from build123d import *

# Parameters (mm, degrees)
SKETCH20_R          = 3.817056353
BOSS_EXTRUDE1_DEPTH = 3.81
BOSS_EXTRUDE2_START = -1.27
BOSS_EXTRUDE2_DEPTH = 1.27
SKETCH23_R          = 2.032
BOSS_EXTRUDE3_DEPTH = 8.636
BOSS_EXTRUDE3_TAPER = 1
SKETCH24_R          = 1.143
CUT_EXTRUDE1_DEPTH  = 9.144
FILLET1_R           = 1.016


with BuildPart() as part:
    # Sketch20 → Boss-Extrude1 (new, symmetric)
    with BuildSketch(Plane.XY):
        with BuildLine():
            ThreePointArc((-2.91972198, 4.764553238), (-1.554108268, 4.783053432), (-0.438429427, 5.570774061))
            ThreePointArc((-0.438429427, 5.570774061), (0, 5.588), (0.438429427, 5.570774061))
            ThreePointArc((0.438429427, 5.570774061), (1.554108268, 4.783053432), (2.91972198, 4.764553238))
            ThreePointArc((2.91972198, 4.764553238), (3.28454399, 4.520786965), (3.629115694, 4.249148536))
            ThreePointArc((3.629115694, 4.249148536), (4.068708268, 2.956089591), (5.162638828, 2.13843502))
            ThreePointArc((5.162638828, 2.13843502), (5.314503813, 1.726786965), (5.433603115, 1.304492693))
            ThreePointArc((5.433603115, 1.304492693), (5.0292, 0), (5.433603115, -1.304492693))
            ThreePointArc((5.433603115, -1.304492693), (5.314503813, -1.726786965), (5.162638828, -2.13843502))
            ThreePointArc((5.162638828, -2.13843502), (4.068708268, -2.956089591), (3.629115694, -4.249148536))
            ThreePointArc((3.629115694, -4.249148536), (3.28454399, -4.520786965), (2.91972198, -4.764553238))
            ThreePointArc((2.91972198, -4.764553238), (1.554108268, -4.783053432), (0.438429427, -5.570774061))
            ThreePointArc((0.438429427, -5.570774061), (0, -5.588), (-0.438429427, -5.570774061))
            ThreePointArc((-0.438429427, -5.570774061), (-1.554108268, -4.783053432), (-2.91972198, -4.764553238))
            ThreePointArc((-2.91972198, -4.764553238), (-3.28454399, -4.520786965), (-3.629115694, -4.249148536))
            ThreePointArc((-3.629115694, -4.249148536), (-4.068708268, -2.956089591), (-5.162638828, -2.13843502))
            ThreePointArc((-5.162638828, -2.13843502), (-5.314503813, -1.726786965), (-5.433603115, -1.304492693))
            ThreePointArc((-5.433603115, -1.304492693), (-5.0292, 0), (-5.433603115, 1.304492693))
            ThreePointArc((-5.433603115, 1.304492693), (-5.314503813, 1.726786965), (-5.162638828, 2.13843502))
            ThreePointArc((-5.162638828, 2.13843502), (-4.068708268, 2.956089591), (-3.629115694, 4.249148536))
            ThreePointArc((-3.629115694, 4.249148536), (-3.28454399, 4.520786965), (-2.91972198, 4.764553238))
        make_face()
        with Locations(Location((0, 0, 0), (0, 0, 180))):
            Circle(SKETCH20_R, mode=Mode.SUBTRACT)
    extrude(amount=BOSS_EXTRUDE1_DEPTH, both=True)

    # Sketch21 → Boss-Extrude2 (add)
    with BuildSketch(Plane(origin=(0, 0, -3.81), x_dir=(-1, 0, 0), z_dir=(0, 0, -1)).offset(BOSS_EXTRUDE2_START)):
        with BuildLine():
            ThreePointArc((3.629115694, 4.249148536), (3.28454399, 4.520786965), (2.91972198, 4.764553238))
            ThreePointArc((2.91972198, 4.764553238), (1.554108268, 4.783053432), (0.438429427, 5.570774061))
            ThreePointArc((0.438429427, 5.570774061), (0, 5.588), (-0.438429427, 5.570774061))
            ThreePointArc((-0.438429427, 5.570774061), (-1.554108268, 4.783053432), (-2.91972198, 4.764553238))
            ThreePointArc((-2.91972198, 4.764553238), (-3.28454399, 4.520786965), (-3.629115694, 4.249148536))
            ThreePointArc((-3.629115694, 4.249148536), (-4.068708268, 2.956089591), (-5.162638828, 2.13843502))
            ThreePointArc((-5.162638828, 2.13843502), (-5.314503813, 1.726786965), (-5.433603115, 1.304492693))
            ThreePointArc((-5.433603115, 1.304492693), (-5.0292, 0), (-5.433603115, -1.304492693))
            ThreePointArc((-5.433603115, -1.304492693), (-5.314503813, -1.726786965), (-5.162638828, -2.13843502))
            ThreePointArc((-5.162638828, -2.13843502), (-4.068708268, -2.956089591), (-3.629115694, -4.249148536))
            ThreePointArc((-3.629115694, -4.249148536), (-3.28454399, -4.520786965), (-2.91972198, -4.764553238))
            ThreePointArc((-2.91972198, -4.764553238), (-1.554108268, -4.783053432), (-0.438429427, -5.570774061))
            ThreePointArc((-0.438429427, -5.570774061), (0, -5.588), (0.438429427, -5.570774061))
            ThreePointArc((0.438429427, -5.570774061), (1.554108268, -4.783053432), (2.91972198, -4.764553238))
            ThreePointArc((2.91972198, -4.764553238), (3.28454399, -4.520786965), (3.629115694, -4.249148536))
            ThreePointArc((3.629115694, -4.249148536), (4.068708268, -2.956089591), (5.162638828, -2.13843502))
            ThreePointArc((5.162638828, -2.13843502), (5.314503813, -1.726786965), (5.433603115, -1.304492693))
            ThreePointArc((5.433603115, -1.304492693), (5.0292, 0), (5.433603115, 1.304492693))
            ThreePointArc((5.433603115, 1.304492693), (5.314503813, 1.726786965), (5.162638828, 2.13843502))
            ThreePointArc((5.162638828, 2.13843502), (4.068708268, 2.956089591), (3.629115694, 4.249148536))
        make_face()
    extrude(amount=BOSS_EXTRUDE2_DEPTH)

    # Sketch23 → Boss-Extrude3 (add)
    with BuildSketch(Plane.XY.offset(-2.54)):
        Circle(SKETCH23_R)
    extrude(amount=BOSS_EXTRUDE3_DEPTH, taper=BOSS_EXTRUDE3_TAPER)

    # Sketch24 → Cut-Extrude1 (cut)
    with BuildSketch(Plane.XY.offset(-3.81)):
        with Locations(Location((0, 0, 0), (0, 0, 180))):
            Circle(SKETCH24_R)
    extrude(amount=CUT_EXTRUDE1_DEPTH, mode=Mode.SUBTRACT)

    # Sketch25 → Cut-Revolve1 (revolve, cut)
    with BuildSketch(Plane(origin=(0, 0, 0), x_dir=(0, 0, -1), z_dir=(1, 0, 0)), mode=Mode.PRIVATE) as cut_revolve1_sk:
        Polygon((2.923053238, 5.588), (3.81, 4.701053238), (3.81, 5.588), align=None)
        Polygon((-3.81, 5.588), (-2.923053238, 5.588), (-3.81, 4.701053238), align=None)
    revolve(cut_revolve1_sk.sketch.rotate(Axis((0, 0, 0), (0, 0, -1)), 90), axis=Axis((0, 0, 0), (0, 0, -1)), mode=Mode.SUBTRACT)

    # Fillet1
    fillet1_edges = [part.edges().sort_by_distance(p)[0] for p in [
        (1.143, 0, -3.81),
    ]]
    fillet(fillet1_edges, radius=FILLET1_R)


solid = part.part
Verification items for the finished model (mm, model axes). A direction names the side the tool comes from. Give positions to 0.01 mm unless a question says otherwise; leave off trailing zeros. Loops run counter-clockwise (first coordinate to the right, second up) from the corner with the lowest first, then second, coordinate; pieces in that order, holes last. Notation, with made-up numbers: (-19.5, 1.25) - (26.5, 1.25) arc R27 cw to (26.5, 18.25) - close; hole circle Ø4 at (18, 62). An arc over 180 degrees is marked (long way). Write item = value, one per line. Start each with the question number.
Q1. Mould release check, pull along Y, two halves, no side actions. Record for faces 4 (the face through (4.62, -1.45, -3.67)), 5 (the face through (-0.527, 1.014, 1.213)), 6 (the face through (-5.313, -1.733, 0.041)): released by +Y, released by -Y, zero draft, split by the parting line, or undercut.
Q2. Depth check by flat-ended pin: P1, Ø1.5, axis at x = 0, y = -3.5, coming from the +Z side; P2, Ø3, axis at x = -3.5, z = -1.5, coming from the -Y side; P3, Ø3, axis at x = 2, z = 1, coming from the -Y side. Enter the tip coordinate at first touch or a pass-through.
Q3. Cross-section at A-A, the plane z = 0.5. Enter the section's corners in (x, y).
Q4. Thickness scan on line 1 (Y direction, x = 1.5, z = 1.5); line 2 (Y direction, x = 0, z = 3.5); line 3 (Z direction, x = -2.25, y = -2.75). Record the ranges inside material, lowest first.
Q5. Tool access check on faces 1 (the face through (-0.42, -1.91, 1.84)), 2 (the face through (-0.006, 5.588, 0.041)), 3 (the face through (0, 0, 5.334)). Record the directions out of +Z, -Z, +X, -X, +Y, -Y that give a thin tool (end or side, any length) a straight path to the whole face; none if there is none.
Q6. Cross-section at B-B, the plane z = 1.5. Enter the section's corners in (x, y).
Answer key:
q1.face_4 = split by the parting line
q1.face_5 = undercut
q1.face_6 = released by -Y
q2.P1 = 3.81
q2.P2 = -4.76
q2.P3 = -5.49
q3.outline = (-5.43, -1.3) arc R5.59 ccw to (-5.16, -2.14) arc R2.31 cw to (-3.63, -4.25) arc R5.59 ccw to (-2.92, -4.76) arc R2.31 cw to (-0.44, -5.57) arc R5.59 ccw to (0.44, -5.57) arc R2.31 cw to (2.92, -4.76) arc R5.59 ccw to (3.63, -4.25) arc R2.31 cw to (5.16, -2.14) arc R5.59 ccw to (5.43, -1.3) arc R2.31 cw to (5.43, 1.3) arc R5.59 ccw to (5.16, 2.14) arc R2.31 cw to (3.63, 4.25) arc R5.59 ccw to (2.92, 4.76) arc R2.31 cw to (0.44, 5.57) arc R5.59 ccw to (-0.44, 5.57) arc R2.31 cw to (-2.92, 4.76) arc R5.59 ccw to (-3.63, 4.25) arc R2.31 cw to (-5.16, 2.14) arc R5.59 ccw to (-5.43, 1.3) arc R2.31 cw to start; circle Ø3.96 at (0, 0); hole circle Ø7.63 at (0, 0); hole circle Ø2.29 at (0, 0)
q4.line_1 = -4.8 to -3.51, -1.26 to 1.26, 3.51 to 4.8
q4.line_2 = -5.01 to -3.82, -1.93 to -1.14, 1.14 to 1.93, 3.82 to 5.01
q4.line_3 = -3.81 to -2.54
q5.face_1 = +Z
q5.face_2 = +Z, -Z, +Y
q5.face_3 = -Z
q6.outline = (-5.43, -1.3) arc R5.59 ccw to (-5.16, -2.14) arc R2.31 cw to (-3.63, -4.25) arc R5.59 ccw to (-2.92, -4.76) arc R2.31 cw to (-0.44, -5.57) arc R5.59 ccw to (0.44, -5.57) arc R2.31 cw to (2.92, -4.76) arc R5.59 ccw to (3.63, -4.25) arc R2.31 cw to (5.16, -2.14) arc R5.59 ccw to (5.43, -1.3) arc R2.31 cw to (5.43, 1.3) arc R5.59 ccw to (5.16, 2.14) arc R2.31 cw to (3.63, 4.25) arc R5.59 ccw to (2.92, 4.76) arc R2.31 cw to (0.44, 5.57) arc R5.59 ccw to (-0.44, 5.57) arc R2.31 cw to (-2.92, 4.76) arc R5.59 ccw to (-3.63, 4.25) arc R2.31 cw to (-5.16, 2.14) arc R5.59 ccw to (-5.43, 1.3) arc R2.31 cw to start; circle Ø3.92 at (0, 0); hole circle Ø7.63 at (0, 0); hole circle Ø2.29 at (0, 0)
